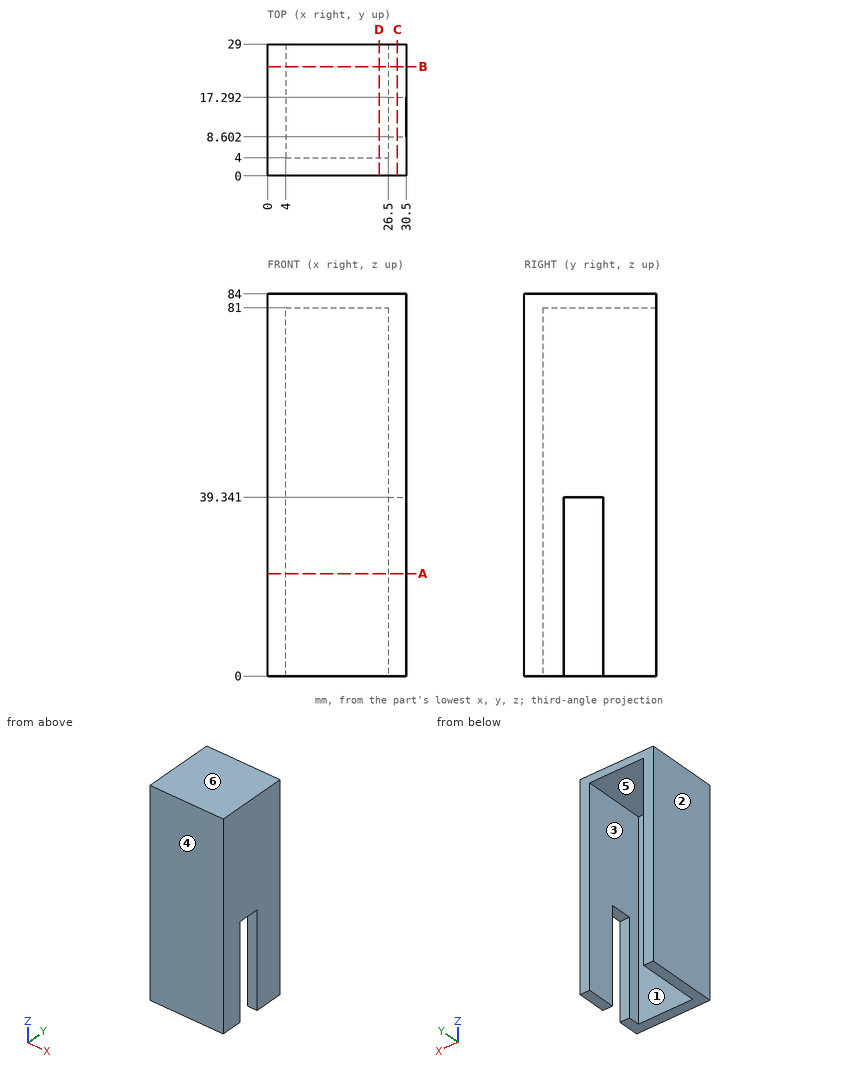
Check sheet for the drawn part. Datum: minimum x, y, z corner. Units: mm. A direction names the side the tool comes from. Round coordinates to 2 decimals unless told otherwise and drop trailing zeros. Order: outer loops, then holes, each group sorted by start corner. A loop starts at its lowest first (then second) coordinate and runs counter-clockwise, first axis right, second up. Notation, with made-up numbers: (82, 71.5) -> (141, 71.5) arc R36 ccw to (141, 109.5) -> close; hole circle Ø6 at (17.5, 7.25). An arc over 180 degrees is marked (long way). Put each result on its own line as item: value. Start each with the question number.
(1) Section check C-C (x = 28.5). Enter the section's corners in (y, z), then the cut area to 3 significant figures.
(2) Section check D-D (x = 24.5). Enter the section's corners in (y, z), then the cut area to 3 significant figures.
(3) Depth check by flat-ended pin: pin 1 Ø2 at (x, z) = (24, 69.5) entering from +Y; pin 2 Ø11 at (x, y) = (19, 11) entering from -Z; pin 3 Ø4.5 at (x, y) = (28, 12.5) entering from -Z. Enter the tip coordinate at first touch or a pass-through.
(4) Section check A-A (z = 22.5). Enter the section's corners in (x, y), then the cut area to 3 significant figures.
(5) Section check B-B (y = 24). Enter the section's corners in (x, z), then the cut area to 4 significant figures.
(6) Tool access check on the marked faces 5 and 6. Record the directions out of +Z, -Z, +X, -X, +Y, -Y that give a thin tool (end or side, any length) a straight path to the whole face; none if there is none.
(7) Draft check along X on the marked faces 1, 2, 3 and 4. Enter one of: +X half, -X half, draft (parallel to the pull), parting line (faces both ways), or undercut.
(8) Material ranges on line 1 along X through (y, z) = (5.75, 43); line 2 along Y through (x, z) = (29, 11); line 3 along Y through (x, z) = (22.5, 53.5), recorded low to high.
Completed:
1. outline: (0, 0) -> (8.6, 0) -> (8.6, 39.34) -> (17.29, 39.34) -> (17.29, 0) -> (29, 0) -> (29, 84) -> (0, 84) -> close
1. area: 2,090 mm2
2. outline: (0, 0) -> (4, 0) -> (4, 81) -> (29, 81) -> (29, 84) -> (0, 84) -> close
2. area: 411 mm2
3. pin 1: stops at y = 4
3. pin 2: stops at z = 81
3. pin 3: stops at z = 39.34
4. outline: (0, 0) -> (30.5, 0) -> (30.5, 8.6) -> (26.5, 8.6) -> (26.5, 4) -> (4, 4) -> (4, 29) -> (0, 29) -> close; (26.5, 17.29) -> (30.5, 17.29) -> (30.5, 29) -> (26.5, 29) -> close
4. area: 287 mm2
5. outline: (0, 0) -> (4, 0) -> (4, 81) -> (26.5, 81) -> (26.5, 0) -> (30.5, 0) -> (30.5, 84) -> (0, 84) -> close
5. area: 739.5 mm2
6. face 5: -Z, +Y
6. face 6: +Z, +X, -X, +Y, -Y
7. face 1: undercut
7. face 2: -X half
7. face 3: undercut
7. face 4: draft
8. line 1: x = 0 to 4, 26.5 to 30.5
8. line 2: y = 0 to 8.6, 17.29 to 29
8. line 3: y = 0 to 4
